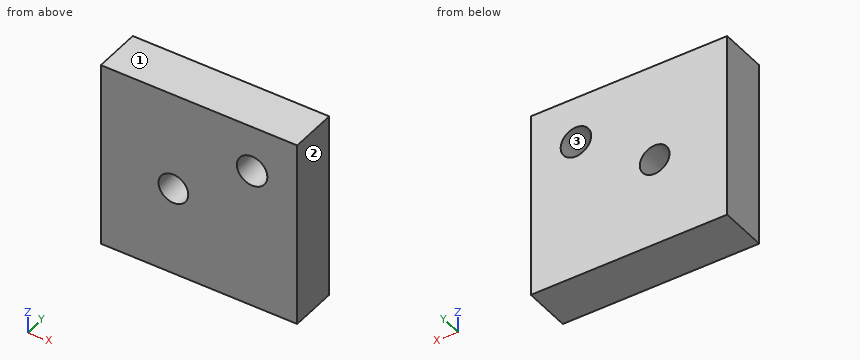
```python
from build123d import *

# Parameters (mm, degrees)
F0_W     = 21.45
F0_H     = 20.45
F1_DEPTH = 5.21
F3_R     = 1.625
F2_R     = 1.665
F4_DEPTH = 5.211


with BuildPart() as f1:
    # F0 (on Front) → F1 (new body)
    with BuildSketch(Plane.XZ):
        Rectangle(F0_W, F0_H)
    extrude(amount=F1_DEPTH)

    # F3 (on face) + F2 (on face) → F4 (cut, through all)
    with BuildSketch(Plane.XZ.offset(5.21)):
        with Locations((-2.8, -0.53)):
            Circle(F3_R)
    with BuildSketch(Plane.XZ.offset(5.21)):
        with Locations((5.8, 5.185)):
            Circle(F2_R)
    extrude(amount=-F4_DEPTH, mode=Mode.SUBTRACT)


solid = f1.part
```
Check sheet for the modelled part. Datum: model origin and axes. Units: mm. Face numbers are marked on the shaded views. Coordinates: 2 decimals unless noted, no trailing zeros. Loops run counter-clockwise (first coordinate to the right, second up) from the corner with the lowest first, then second, coordinate; pieces in that order, holes last.
1) Material ranges on probe 1 along Z at (x, y) = (5.8, -2.3) (3 decimals); probe 2 along Z at (x, y) = (-2.8, -3.3) (3 decimals); probe 3 along X at (y, z) = (-3.85, 5.5) (3 decimals), recorded low to high.
2) Sectioned sample at A-A (z = -0.53). Record the boundary of the cut face in (x, y) (3 decimals).
3) Sectioned sample at C-C (y = -0.7). Record the boundary of the cut face in (x, z) (3 decimals).
4) Release check for a two-part mould opening along X. For the marked faces 1, 2 and 3 record: released by +X, released by -X, zero draft, split by the parting line, or undercut.
5) Gauge pin test, flat end, axial feed: pin 1 (2.5 mm diameter, centred on x = 5.8, z = 5.185, fed in from -Y). Record the tip position at first contact, or that the pin passes through.
6) Sectioned sample at B-B (x = 5.8). Record the boundary of the cut face in (y, z) (3 decimals), and give its area (3 significant figures).
Check sheet entries:
1. probe 1: z = -10.225 to 3.52, 6.85 to 10.225
1. probe 2: z = -10.225 to -2.155, 1.095 to 10.225
1. probe 3: x = -10.725 to 4.165, 7.435 to 10.725
2. outline: (-10.725, -5.21) - (-4.425, -5.21) - (-4.425, 0) - (-10.725, 0) - close; (-1.175, -5.21) - (10.725, -5.21) - (10.725, 0) - (-1.175, 0) - close
3. outline: (-10.725, -10.225) - (10.725, -10.225) - (10.725, 10.225) - (-10.725, 10.225) - close; hole circle Ø3.25 at (-2.8, -0.53); hole circle Ø3.33 at (5.8, 5.185)
4. face 1: zero draft
4. face 2: released by +X
4. face 3: undercut
5. pin 1: passes through
6. outline: (-5.21, -10.225) - (0, -10.225) - (0, 3.52) - (-5.21, 3.52) - close; (-5.21, 6.85) - (0, 6.85) - (0, 10.225) - (-5.21, 10.225) - close
6. area: 89.2 mm2
